```python
from build123d import *

# Parameters (mm, degrees)
SKETCH_W      = 20
SKETCH_H      = 4
EXTRUDE_DEPTH = 10


with BuildPart() as part:
    # Sketch → Extrude (new body)
    with BuildSketch(Plane.XY):
        Polygon((28.867513, 0), (14.433757, 25), (-14.433757, 25), (-28.867513, 0), (-14.433757, -25), (14.433757, -25), align=None)
        Polygon((7.5, 23.082627), (-7.5, 23.082627), (-12.135255, 8.816779), (0, 0), (12.135255, 8.816779), align=None, mode=Mode.SUBTRACT)
        with Locations((0, -17)):
            Rectangle(SKETCH_W, SKETCH_H, mode=Mode.SUBTRACT)
    extrude(amount=EXTRUDE_DEPTH)


solid = part.part
```
Can you work these out from the model? Positions are in its coordinate system, mm. A direction names the side the tool comes from. Round coordinates to 2 decimals unless told otherwise and drop trailing zeros. Order: outer loops, then holes, each group sorted by start corner. A loop starts at its lowest first (then second) coordinate and runs counter-clockwise, first axis right, second up. Notation, with made-up numbers: (53, 8) -> (107, 8) arc R27 ccw to (107, 27) -> close; hole circle Ø9 at (-2, -30). An arc over 180 degrees is marked (long way). Return JSON: item names as keys, results as strings. Group by question number.
1. If we section it at D-D, the plane y = 11: Write out the boundary of the cut face in (x, z), then the cut area to 3 significant figures.
2. We'd pull the mould along X, two halves only. Please class faces 3 (the face through (-21.55, 12.675, 4.93)), 4 (the face through (9.85, 15.85, 4.93)), 5 (the face through (21.55, -12.675, 4.93)): released by +X, released by -X, zero draft, split by the parting line, or undercut.
3. If we section it at B-B, the plane z = 7.25: Write out the boundary of the cut face in (x, y), then the cut area to 3 significant figures.
4. Which directions (+Z, -Z, +X, -X, +Y, -Y) give clear straight access to the entire face, cutting with the end or side of a thin tool? Please do faces 1 (the face through (10, -17, 5)), 2 (the face through (-21.752, -12.325, 4.93)).
5. I need wall thicknesses on line 1 (Y direction, x = -1.5, z = 5.5); line 2 (Y direction, x = -2, z = 5.75); line 3 (X direction, y = 2.5, z = 2.75). Which ranges of each line are inside material? Lowest first, please. Write a range as [from, to].
6. If we section it at A-A, the plane y = 18: Write out the boundary of the cut face in (x, z).
7. If we section it at C-C, the plane x = -4: Write out the boundary of the cut face in (y, z), then the cut area to 3 significant figures.
8. Will these pins go through, and if not, where does the flat tip stop? pin 1 (4 mm diameter, centred on x = 16.5, z = 8, fed in from -Y); pin 2 (5 mm diameter, centred on y = -12.5, z = 7, fed in from -X); pin 3 (4.5 mm diameter, centred on y = -17.5, z = 3.5, fed in from +X).
Output values:
{
 "1": {"outline": "(-22.52, 0) -> (-11.43, 0) -> (-11.43, 10) -> (-22.52, 10) -> close; (11.43, 0) -> (22.52, 0) -> (22.52, 10) -> (11.43, 10) -> close", "area": "222 mm²"},
 "2": {"face 3": "released by -X", "face 4": "undercut", "face 5": "released by +X"},
 "3": {"outline": "(-28.87, 0) -> (-14.43, -25) -> (14.43, -25) -> (28.87, 0) -> (14.43, 25) -> (-14.43, 25) -> close; hole (-12.14, 8.82) -> (0, 0) -> (12.14, 8.82) -> (7.5, 23.08) -> (-7.5, 23.08) -> close; hole (-10, -19) -> (10, -19) -> (10, -15) -> (-10, -15) -> close", "area": "1,700 mm²"},
 "4": {"face 1": "+Z, -Z", "face 2": "+Z, -Z, -X, -Y"},
 "5": {"line 1": "[-25, -19], [-15, 1.09], [23.08, 25]", "line 2": "[-25, -19], [-15, 1.45], [23.08, 25]", "line 3": "[-27.42, -3.44], [3.44, 27.42]"},
 "6": {"outline": "(-18.48, 0) -> (-9.15, 0) -> (-9.15, 10) -> (-18.48, 10) -> close; (9.15, 0) -> (18.48, 0) -> (18.48, 10) -> (9.15, 10) -> close"},
 "7": {"outline": "(-25, 0) -> (-19, 0) -> (-19, 10) -> (-25, 10) -> close; (-15, 0) -> (2.91, 0) -> (2.91, 10) -> (-15, 10) -> close; (23.08, 0) -> (25, 0) -> (25, 10) -> (23.08, 10) -> close", "area": "258 mm²"},
 "8": {"pin 1": "y = -24.89", "pin 2": "x = -23.09", "pin 3": "x = 20.06"}
}
